Input: dimensioned drawing with shaded views. Units: mm. Origin: part minimum x, y, z. Coordinates: 2 decimals unless noted, no trailing zeros. Order: outer loops, then holes, each group sorted by start corner. A loop starts at its lowest first (then second) coordinate and runs counter-clockwise, first axis right, second up. Notation, with made-up numbers: (38.25, -9) - (60.25, -9) arc R15 cw to (60.25, 12) - close; hole circle Ø7 at (-30.75, 61). An arc over 180 degrees is marked (long way). Answer as CSV lines item,"result". Start each with the question number.
Item 1: First-contact query: pin 1 (6 mm diameter, centred on x = 14, y = 11, fed in from +Z); pin 2 (1.9 mm diameter, centred on x = 19, y = 16.25, fed in from +Z). Flat tips, straight axial feed; report the tip coordinate or a pass-through.
Item 2: Draft query along Y for the marked faces 1 and 2. Return one class per face: +Y half, -Y half, draft (parallel to the pull), parting line (faces both ways), or undercut.
Item 3: Section C-C (x = 19.25). Output: boundary loops of the cut face in (y, z).
Item 4: Section B-B (x = 12.5). Output: boundary loops of the cut face in (y, z), and give its area (3 significant figures).
Item 5: Material intervals for line 1 along Y through (x, z) = (12.5, 0.4); line 2 along Y through (x, z) = (12.5, 1); line 3 along Z through (x, y) = (15.5, 15.25), sorted ascending.
Item 6: Section D-D (z = 0.65). State how many separate pieces and enclosed holes the cut face has, and give its area (3 significant figures).
Item 7: Section A-A (y = 5). Output: boundary loops of the cut face in (x, z).
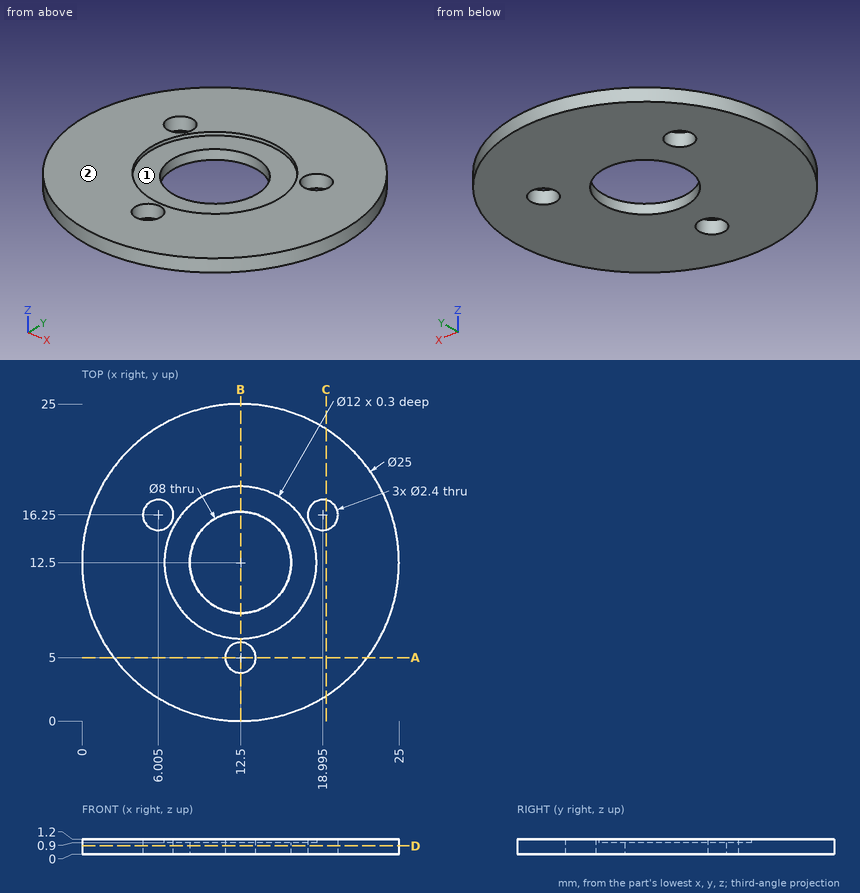
Determined:
1,pin 1,"stops at z = 0.9"
1,pin 2,"passes through"
2,face 1,"undercut"
2,face 2,"draft"
3,outline,"(1.98, 0) - (15.08, 0) - (15.08, 1.2) - (1.98, 1.2) - close; (17.42, 0) - (23.02, 0) - (23.02, 1.2) - (17.42, 1.2) - close"
4,outline,"(0, 0) - (3.8, 0) - (3.8, 1.2) - (0, 1.2) - close; (6.2, 0) - (8.5, 0) - (8.5, 0.9) - (6.5, 0.9) - (6.5, 1.2) - (6.2, 1.2) - close; (16.5, 0) - (25, 0) - (25, 1.2) - (18.5, 1.2) - (18.5, 0.9) - (16.5, 0.9) - close"
4,area,"16.3 mm^2"
5,line 1,"y = 0 to 3.8, 6.2 to 8.5, 16.5 to 25"
5,line 2,"y = 0 to 3.8, 6.2 to 6.5, 18.5 to 25"
5,line 3,"z = 0 to 0.9"
6,separate pieces,"1"
6,enclosed holes,"4"
6,area,"427 mm^2"
7,outline,"(2.5, 0) - (11.3, 0) - (11.3, 1.2) - (2.5, 1.2) - close; (13.7, 0) - (22.5, 0) - (22.5, 1.2) - (13.7, 1.2) - close"
